```python
from build123d import *

# Parameters (mm, degrees)
BOSS_EXTRUDE1_DEPTH = 2
PCBLEDGE_DEPTH      = 3
BOSS_EXTRUDE3_DEPTH = 5
SKETCH4_R           = 1.5
FORSCREWS_DEPTH     = 2
GROOVE_DEPTH        = 2
SKETCH6_W           = 5
SKETCH6_H           = 8
BOSS_EXTRUDE6_DEPTH = 8
CUT_EXTRUDE1_DEPTH  = 7


with BuildPart() as part:
    # Sketch1 → Boss-Extrude1 (new body)
    with BuildSketch(Plane(origin=(0, 0, 0), x_dir=(1, 0, 0), z_dir=(0, 1, 0))):
        Polygon((-7, 12.5), (-23, 12.5), (-25, 10.5), (-25, -10.5), (-23, -12.5), (23, -12.5), (25, -10.5), (25, 10.5), (23, 12.5), (7, 12.5), (7, 8.5), (5, 6.5), (-5, 6.5), (-7, 8.5), align=None)
    extrude(amount=BOSS_EXTRUDE1_DEPTH)

    # Sketch2 → PcbLedge (add)
    with BuildSketch(Plane(origin=(0, 2, 0), x_dir=(1, 0, 0), z_dir=(0, 1, 0))):
        with BuildLine():
            Line((23, -10.5), (23, -7))
            Line((23, -7), (21, -7))
            ThreePointArc((21, -7), (19.762563133, -7.512563133), (19.25, -8.75))
            Line((19.25, -8.75), (19.25, -10.5))
            Line((19.25, -10.5), (23, -10.5))
        make_face()
        with BuildLine():
            Line((23, 10.5), (19.25, 10.5))
            Line((19.25, 10.5), (19.25, 8.75))
            ThreePointArc((19.25, 8.75), (19.762563133, 7.512563133), (21, 7))
            Line((21, 7), (23, 7))
            Line((23, 7), (23, 10.5))
        make_face()
        with BuildLine():
            Line((-19.25, 8.75), (-19.25, 10.5))
            Line((-19.25, 10.5), (-23, 10.5))
            Line((-23, 10.5), (-23, 7))
            Line((-23, 7), (-21, 7))
            ThreePointArc((-21, 7), (-19.762563133, 7.512563133), (-19.25, 8.75))
        make_face()
        with BuildLine():
            Line((-23, -10.5), (-19.25, -10.5))
            Line((-19.25, -10.5), (-19.25, -8.75))
            ThreePointArc((-19.25, -8.75), (-19.762563133, -7.512563133), (-21, -7))
            Line((-21, -7), (-23, -7))
            Line((-23, -7), (-23, -10.5))
        make_face()
    extrude(amount=PCBLEDGE_DEPTH)

    # Sketch2_3 → Boss-Extrude3 (add)
    with BuildSketch(Plane(origin=(0, 2, 0), x_dir=(1, 0, 0), z_dir=(0, 1, 0))):
        Polygon((7, 12.5), (23, 12.5), (25, 10.5), (25, -10.5), (23, -12.5), (0, -12.5), (-23, -12.5), (-25, -10.5), (-25, 10.5), (-23, 12.5), (-7, 12.5), (-7, 10.5), (-23, 10.5), (-23, -10.5), (0, -10.5), (23, -10.5), (23, 10.5), (7, 10.5), align=None)
    extrude(amount=BOSS_EXTRUDE3_DEPTH)

    # Sketch4 → ForScrews (add)
    # profile 1 of 2: a face of its own
    with BuildSketch(Plane.XZ):
        Polygon((21, -12.5), (17.5, -19.5), (12.5, -19.5), (9, -12.5), align=None)
        with Locations(Location((15, -16, 0), (0, 0, 270))):
            Circle(SKETCH4_R, mode=Mode.SUBTRACT)
    # profile 2 of 2: a face of its own
    with BuildSketch(Plane.XZ):
        Polygon((-12.5, 19.5), (-9, 12.5), (-21, 12.5), (-17.5, 19.5), align=None)
        with Locations(Location((-15, 16, 0), (0, 0, 270))):
            Circle(SKETCH4_R, mode=Mode.SUBTRACT)
    extrude(amount=-FORSCREWS_DEPTH)

    # Sketch5 → Groove (add)
    with BuildSketch(Plane(origin=(0, 7, 0), x_dir=(1, 0, 0), z_dir=(0, 1, 0))):
        Polygon((25, 10.5), (23, 12.5), (7, 12.5), (7, 11.5), (22.585786438, 11.5), (24, 10.085786438), (24, -10.085786438), (22.585786438, -11.5), (-22.585786438, -11.5), (-24, -10.085786438), (-24, 10.085786438), (-22.585786438, 11.5), (-7, 11.5), (-7, 12.5), (-23, 12.5), (-25, 10.5), (-25, -10.5), (-23, -12.5), (23, -12.5), (25, -10.5), align=None)
    extrude(amount=GROOVE_DEPTH)

    # Sketch6 → Boss-Extrude6 (add)
    with BuildSketch(Plane.XZ):
        with Locations((-16.5, -16.5)):
            Rectangle(SKETCH6_W, SKETCH6_H)
    extrude(amount=-BOSS_EXTRUDE6_DEPTH)

    # Sketch7 → Cut-Extrude1 (cut)
    with BuildSketch(Plane.ZY.offset(19)):
        with BuildLine():
            Line((-16.5, 2), (-12.5, 2))
            Line((-12.5, 2), (-12.5, 8.728396631))
            Line((-12.5, 8.728396631), (-18.5, 8.728396631))
            Line((-18.5, 8.728396631), (-18.5, 4))
            ThreePointArc((-18.5, 4), (-17.914213562, 2.585786438), (-16.5, 2))
        make_face()
    extrude(amount=-CUT_EXTRUDE1_DEPTH, mode=Mode.SUBTRACT)


solid = part.part
```
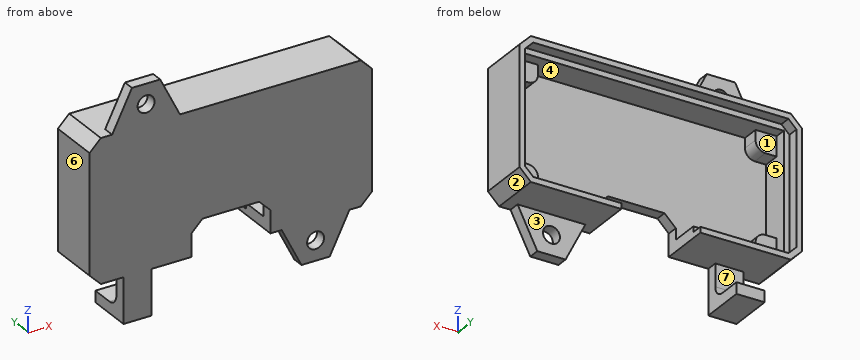
The model under review builds one solid part; all positions refer to its coordinate system, in mm. Face numbers are marked on the shaded views. A direction names the side the tool comes from. Round coordinates to 2 decimals unless told otherwise and drop trailing zeros. Loops run counter-clockwise (first coordinate to the right, second up) from the corner with the lowest first, then second, coordinate; pieces in that order, holes last. Notation, with made-up numbers: (24.25, 24.25) - (46.25, 24.25) arc R24 ccw to (46.25, 54.25) - close; hole circle Ø10 at (61, 40). An arc over 180 degrees is marked (long way). Use a Markdown table: item, result. Add a question column.
Q1. Insertion check: pin 1 Ø3.5 at (x, z) = (-14.5, 15.5) entering from +Y; pin 2 Ø4 at (x, y) = (-5.5, 2.5) entering from -Z; pin 3 Ø2.5 at (x, z) = (-15, 16) entering from -Y; pin 4 Ø1.5 at (x, y) = (6.5, 1) entering from +Z. Each pin has a flat end and moves straight along its axis. Give the tip position at first contact, or say it passes through.
Q2. Add section C-C (y = 6.25). State the section outline as (x, z) points.
Q3. Machinability: for the marked faces 1, 2 and 3, which of the approach directions +Z, -Z, +X, -X, +Y, -Y give a long, thin tool a straight path to every point of the face, cutting with its end or side? Answer none if there is none.
Q4. Add section D-D (z = -1). State the section outline as (x, y) points.
Q5. The part is to be moulded in two halves that separate along X. For the marked faces 4, 5, 6 and 7, say which applies: pulls with the +X half, pulls with the -X half, needs draft (parallel to the pull), parting line crosses it, or undercut.
Q6. Add section B-B (x = 15). State the section outline as (y, z) points.
Q7. For probe 1 along X at (y, z) = (7.25, 6.5); probe 2 along Z at (x, y) = (9.5, 3.5); probe 3 along X at (y, z) = (1.55, -16), list the stretches that pass through material, from the lowest coordinate up.
Q8. Add section A-A (z = 16). State the section outline as (x, y) points, plus the area to 3 significant figures.
Worked answers:
| question | item | result |
|---|---|---|
| 1 | pin 1 | y = 2 |
| 1 | pin 2 | z = -12.5 |
| 1 | pin 3 | through |
| 1 | pin 4 | z = 12.5 |
| 2 | outline | (-25, -10.5) - (-23, -12.5) - (-7, -12.5) - (-7, -10.5) - (-23, -10.5) - (-23, 10.5) - (23, 10.5) - (23, -10.5) - (7, -10.5) - (7, -12.5) - (23, -12.5) - (25, -10.5) - (25, 10.5) - (23, 12.5) - (-23, 12.5) - (-25, 10.5) - close; (-19, -20.5) - (-14, -20.5) - (-14, -18.5) - (-19, -18.5) - close |
| 3 | face 1 | +Y |
| 3 | face 2 | -Z, +X, +Y, -Y |
| 3 | face 3 | -Z, +X, +Y |
| 4 | outline | (-25, 0) - (25, 0) - (25, 9) - (24, 9) - (24, 7) - (23, 7) - (23, 2) - (-23, 2) - (-23, 7) - (-24, 7) - (-24, 9) - (-25, 9) - close |
| 5 | face 4 | undercut |
| 5 | face 5 | undercut |
| 5 | face 6 | pulls with the -X half |
| 5 | face 7 | needs draft |
| 6 | outline | (0, -19.5) - (2, -19.5) - (2, -17.5) - (0, -17.5) - close; (0, -14.5) - (2, -14.5) - (2, -12.5) - (9, -12.5) - (9, -11.5) - (7, -11.5) - (7, -10.5) - (2, -10.5) - (2, 10.5) - (7, 10.5) - (7, 11.5) - (9, 11.5) - (9, 12.5) - (0, 12.5) - close |
| 7 | probe 1 | -25 to -24, 24 to 25 |
| 7 | probe 2 | -12.5 to -10.5, 10.5 to 12.5 |
| 7 | probe 3 | -19 to -14, 10.75 to 13.5, 16.5 to 19.25 |
| 8 | outline | (-19.25, 0) - (-16.5, 0) - (-16.5, 2) - (-19.25, 2) - close; (-13.5, 0) - (-10.75, 0) - (-10.75, 2) - (-13.5, 2) - close |
| 8 | area | 11.0 mm² |
